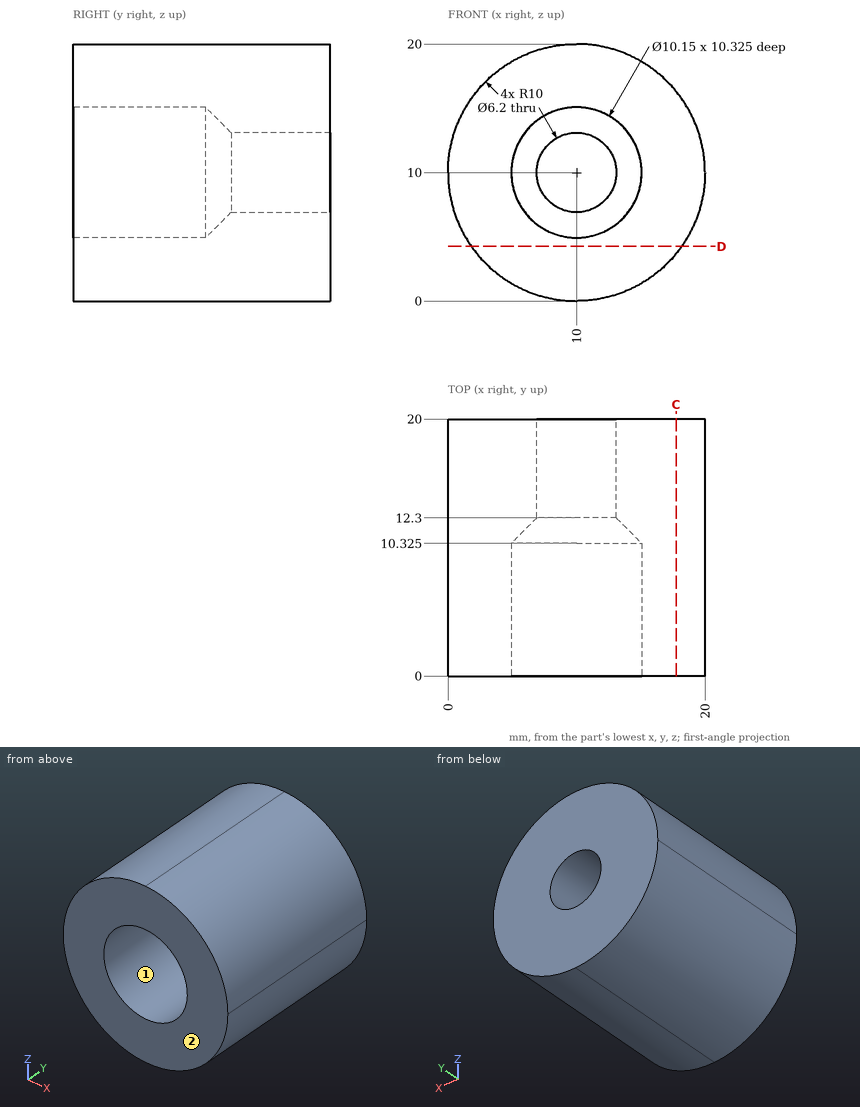
Here's the drawing with two shaded views (mm, measured from the low corner). I have some questions. A direction names the side the tool comes from. Round coordinates to 2 decimals unless told otherwise and drop trailing zeros. Write each loop counter-clockwise with the first axis right and the second up, starting at its lowest first coordinate (ties: lowest second). Pieces come first, ordered by that corner, then holes. Notation, with made-up numbers: M -39,-36.5 L 6,-36.5 A10 cw 6,-30.5 Z; hole C 29,-12 d3. An arc over 180 degrees is marked long. Answer in a Markdown table with one row per item. Add a question column.
Q1. If I drill on line 1 (X direction, y = 4.5, z = 10) (3 decimals); line 2 (X direction, y = 16.5, z = 10); line 3 (Z direction, x = 6.75, y = 6.5), over which ranges is the centre line in solid material (lowest first)? Write a range as from..to.
Q2. Imagine slicing it at C-C (x = 17.75). Please give me the cut outline in (y, z).
Q3. Imagine slicing it at D-D (z = 4.25). Please give me the cut outline in (x, y).
Q4. Will these pins go through, and if not, where does the flat tip stop? pin 1 Ø6 at (x, z) = (10, 10) entering from -Y; pin 2 Ø8 at (x, y) = (3.5, 16) entering from -Z; pin 3 Ø8 at (y, z) = (2.5, 17.5) entering from -X; pin 4 Ø8 at (x, z) = (10, 10) entering from -Y.
Q5. On a 3-axis mill with a long thin cutter (end or side, diameter ignored), from which of +Z, -Z, +X, -X, +Y, -Y can I reach the whole of each face in a straight line? I mean the marked faces 1 and 2. Say none if no direction works.
Values:
| question | item | result |
|---|---|---|
| 1 | line 1 | 0..4.925, 15.075..20 |
| 1 | line 2 | 0..6.9, 13.1..20 |
| 1 | line 3 | 0.54..6.1, 13.9..19.46 |
| 2 | outline | M 0,3.68 L 20,3.68 L 20,16.32 L 0,16.32 Z |
| 3 | outline | M 1.82,0 L 18.18,0 L 18.18,20 L 1.82,20 Z |
| 4 | pin 1 | through |
| 4 | pin 2 | z = 0.32 |
| 4 | pin 3 | x = 0.63 |
| 4 | pin 4 | y = 11.4 |
| 5 | face 1 | -Y |
| 5 | face 2 | +Z, -Z, +X, -X, -Y |
